Geometry: see drawing. Coordinates: mm, zero at the bounding-box minimum. A direction names the side the tool comes from. Coordinates: 2 decimals unless noted, no trailing zeros. Order: outer loops, then holes, each group sorted by start corner. A loop starts at its lowest first (then second) coordinate and runs counter-clockwise, first axis right, second up. Notation, with made-up numbers: (78.5, -18) -> (112.5, -18) arc R22 ccw to (112.5, -9) -> close; hole circle Ø1 at (-2, 29). An arc over 180 degrees is marked (long way). Use one line per item in the form item = value.
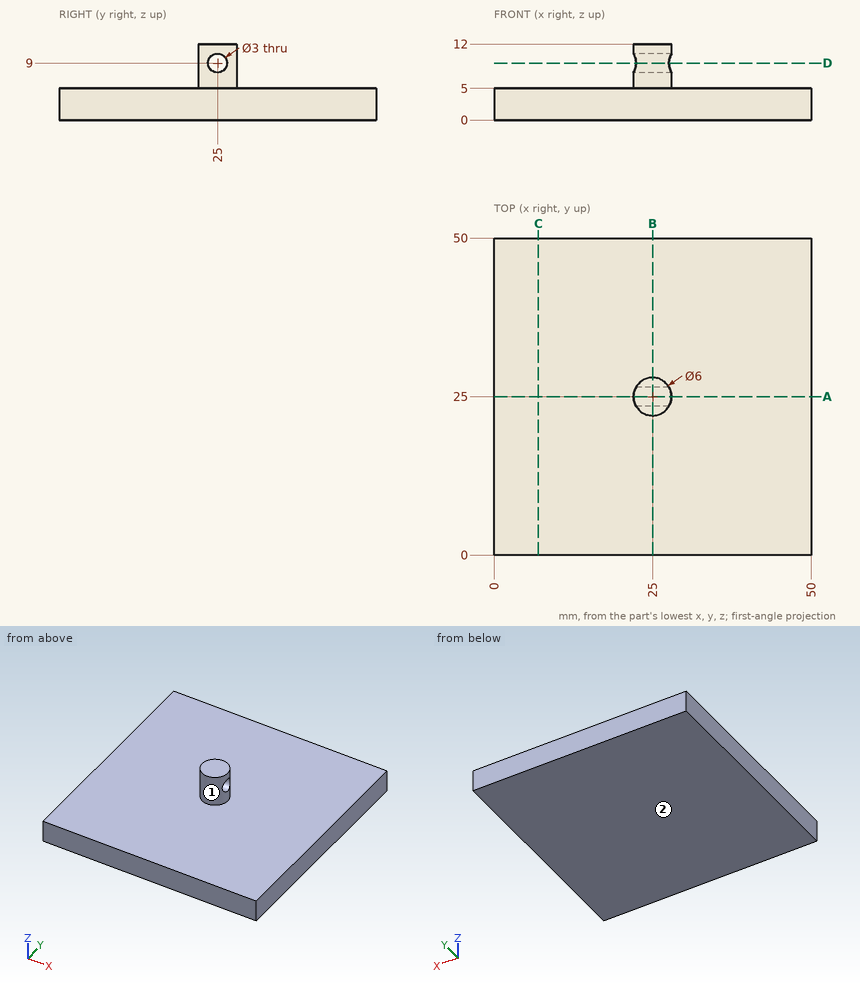
1) Access query for the marked faces 1 and 2. Directions: +Z, -Z, +X, -X, +Y, -Y. A direction counts if a zero-diameter tool reaches every point of the face in a straight line with its end or side. Return the directions, or none.
Results found:
face_1 = +Z
face_2 = -Z, +X, -X, +Y, -Y
2) Section A-A, the plane y = 25. Output: boundary loops of the cut face in (x, z).
Results found:
outline = (0, 0) -> (50, 0) -> (50, 5) -> (28, 5) -> (28, 7.5) -> (22, 7.5) -> (22, 5) -> (0, 5) -> close; (22, 10.5) -> (28, 10.5) -> (28, 12) -> (22, 12) -> close
3) Contact query for flat-ended pins moving along their axis: P1, Ø5, axis at y = 10.5, z = 8.5, coming from the -X side; P2, Ø15, axis at x = 18.5, y = 13, coming from the +Z side. Output: stop coordinate, or through.
Results found:
P1 = through
P2 = 5
4) Section B-B, the plane x = 25. Output: boundary loops of the cut face in (y, z), and give its area (3 significant figures).
Results found:
outline = (0, 0) -> (50, 0) -> (50, 5) -> (28, 5) -> (28, 12) -> (22, 12) -> (22, 5) -> (0, 5) -> close; hole circle Ø3 at (25, 9)
area = 285 mm2
5) Material intervals for probe 1 along Z at (x, y) = (26, 25); probe 2 along Y at (x, z) = (23.5, 9); probe 3 along Z at (x, y) = (30.5, 28.5), sorted ascending. Write a range as from..to.
Results found:
probe_1 = 0..7.5, 10.5..12
probe_2 = 22.4..23.5, 26.5..27.6
probe_3 = 0..5
6) Section C-C, the plane x = 7. Output: boundary loops of the cut face in (y, z).
Results found:
outline = (0, 0) -> (50, 0) -> (50, 5) -> (0, 5) -> close
7) Section D-D, the plane z = 9. Output: boundary loops of the cut face in (x, y).
Results found:
outline = (22.4, 23.5) arc R3 ccw to (27.6, 23.5) -> close; (22.4, 26.5) -> (27.6, 26.5) arc R3 ccw to start
